```python
from build123d import *

# Parameters (mm, degrees)
F0_W     = 172
F0_H     = 172
F1_DEPTH = 50
F2_W     = 162
F2_H     = 162
F2_W_2   = 122
F2_H_2   = 122
F3_DEPTH = 45
F4_T     = -2.5
F5_R     = 5
F6_DEPTH = 9.5


# Not quite as in the source:
# - a shell that OpenCascade refuses in one call is made with other operations: the cavity is built on its own and cut out


with BuildPart() as f1:
    # F0 (on Top) → F1 (new body)
    with BuildSketch(Plane.XY):
        Rectangle(F0_W, F0_H)
    extrude(amount=F1_DEPTH)

    # F2 (on Top) → F3 (cut)
    with BuildSketch(Plane.XY):
        Rectangle(F2_W, F2_H)
        Rectangle(F2_W_2, F2_H_2, mode=Mode.SUBTRACT)
    extrude(amount=F3_DEPTH, mode=Mode.SUBTRACT)

    # F4: a shell. OpenCascade refuses it in one call, so the cavity is built on its own and cut out:
    # the body offset inwards by the wall thickness, plus a prism from it out through each open face.
    f4_core = offset(f1.part, amount=F4_T, kind=Kind.INTERSECTION, mode=Mode.PRIVATE)
    f4_exits = [f4_core.faces().sort_by_distance(p)[0] for p in [
        (0, 0, 2.5),
    ]]
    add(f4_core, mode=Mode.SUBTRACT)
    extrude(f4_exits, amount=-F4_T, mode=Mode.SUBTRACT)

    # F5 (on face) → F6 (cut)
    with BuildSketch(Plane(origin=(0, 86, 0), x_dir=(-1, 0, 0), z_dir=(0, 1, 0))):
        with Locations((42.7398793399, 25)):
            Circle(F5_R)
        with Locations((-42.7398793399, 25)):
            Circle(F5_R)
    extrude(amount=-F6_DEPTH, mode=Mode.SUBTRACT)


solid = f1.part
```
Geometry: final body of the model. Coordinates: model frame, mm. A direction names the side the tool comes from. Coordinates: 2 decimals unless noted, no trailing zeros. Order: outer loops, then holes, each group sorted by start corner. A loop starts at its lowest first (then second) coordinate and runs counter-clockwise, first axis right, second up. Notation, with made-up numbers: M -8.5,22.5 L 10.5,22.5 A8 ccw 10.5,26.5 Z; hole C 39,43 d6. An arc over 180 degrees is marked long. Answer in a Markdown table with one row per item. Add a question column.
Q1. Reachability of faces 5 (the flat face through (-1, -58.5, 24)), 6 (the cylindrical face through (43.82, 83.54, 20.12)), 7 (the flat face through (-1, 1, 50)) from +Z, -Z, +X, -X, +Y, -Y: full face, straight path, thin tool, end or side. Return the list, or none.
Q2. Mould query, pull axis X, two halves, no side actions, for faces 1 (the flat face through (-7, -82, 0)), 2 (the cylindrical face through (-45.047, 83.535, 20.564)), 3 (the flat face through (-86, -1, 25)), 4 (the flat face through (81, -1, 22)). Classes: released by +X, released by -X, zero draft, split by the parting line, or undercut.
Q3. Section query A-A on z = 25. Return the cut outline in (x, y), and give its area (4 significant figures).
Q4. Line query: L1, parallel to X at y = 43.5, z = 6.5; L2, parallel to Y at x = -42, z = 25.5. Output: solid intervals per line, ascending.
Q5. Contact query for a flat-ended pin moving along its axis: P1, Ø5, axis at x = -37, y = 4, coming from the -Z side. Output: stop coordinate, or through.
Q6. Section query D-D on y = 75. Return the cut outline in (x, z), and give its area (3 significant figures).
Q7. Section query B-B on y = -5. Return the cut outline in (x, z), and give its area (3 significant figures).
Completed:
| question | item | result |
|---|---|---|
| 1 | face 5 | -Z |
| 1 | face 6 | +Y |
| 1 | face 7 | +Z, +X, -X, +Y, -Y |
| 2 | face 1 | zero draft |
| 2 | face 2 | undercut |
| 2 | face 3 | released by -X |
| 2 | face 4 | undercut |
| 3 | outline | M -86,-86 L 86,-86 L 86,86 L 47.74,86 L 47.74,81 L 81,81 L 81,-81 L -81,-81 L -81,81 L -47.74,81 L -47.74,86 L -86,86 Z; M -61,-61 L 61,-61 L 61,61 L -61,61 Z; M -37.74,81 L 37.74,81 L 37.74,86 L -37.74,86 Z; hole M -58.5,-58.5 L 58.5,-58.5 L 58.5,58.5 L -58.5,58.5 Z |
| 3 | area | 4,435 mm2 |
| 4 | L1 | x = -86 to -81, -61 to -58.5, 58.5 to 61, 81 to 86 |
| 4 | L2 | y = -86 to -81, -61 to -58.5, 58.5 to 61 |
| 5 | P1 | stops at z = 47.5 |
| 6 | outline | M -86,0 L -81,0 L -81,45 L 81,45 L 81,0 L 86,0 L 86,50 L -86,50 Z |
| 6 | area | 1,310 mm2 |
| 7 | outline | M -86,0 L -81,0 L -81,45 L -61,45 L -61,0 L -58.5,0 L -58.5,47.5 L 58.5,47.5 L 58.5,0 L 61,0 L 61,45 L 81,45 L 81,0 L 86,0 L 86,50 L -86,50 Z |
| 7 | area | 1,240 mm2 |
